Here's how the part is built. I have some questions about the finished solid (model axes, mm). Face numbers are marked on the shaded views. A direction names the side the tool comes from. Give positions to 0.01 mm unless a question says otherwise; leave off trailing zeros. Write each loop counter-clockwise with the first axis right and the second up, starting at its lowest first coordinate (ties: lowest second). Pieces come first, ordered by that corner, then holes. Notation, with made-up numbers: (76.5, 50) -> (127.5, 50) arc R25 ccw to (127.5, 84) -> close; hole circle Ø5 at (16.25, 58). An arc over 180 degrees is marked (long way). Use one line per item in the form item = value.
```python
from build123d import *

# Parameters (mm, degrees)
BOSS_EXTRUDE1_DEPTH = 3
SKETCH2_R           = 1.7
CUT_EXTRUDE1_DEPTH  = 3


with BuildPart() as part:
    # Sketch1 → Boss-Extrude1 (new body)
    with BuildSketch(Plane.XY):
        Polygon((10.5, 20.853495779), (-10.5, 20.853495779), (-10.5, 16.353495779), (-5.75, 16.353495779), (-5.75, -11.146504221), (5.75, -11.146504221), (5.75, 16.353495779), (10.5, 16.353495779), align=None)
    extrude(amount=BOSS_EXTRUDE1_DEPTH)

    # Sketch2 → Cut-Extrude1 (cut)
    with BuildSketch(Plane.XY.offset(3)):
        with Locations((0, -6.446504221)):
            Circle(SKETCH2_R)
        with BuildLine():
            Line((1.725328859, 12.62816692), (1.725328859, 9.078824638))
            ThreePointArc((1.725328859, 9.078824638), (0, 7.353495779), (-1.725328859, 9.078824638))
            Line((-1.725328859, 9.078824638), (-1.725328859, 12.62816692))
            ThreePointArc((-1.725328859, 12.62816692), (0, 14.353495779), (1.725328859, 12.62816692))
        make_face()
    extrude(amount=-CUT_EXTRUDE1_DEPTH, mode=Mode.SUBTRACT)


solid = part.part
```
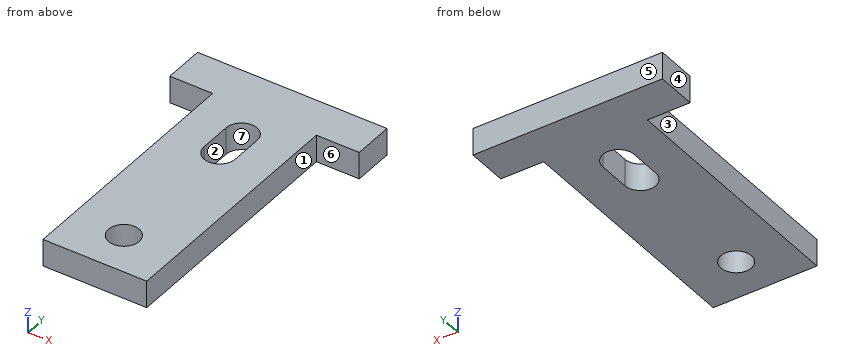
Q1. If I drill on line 1 along Y through (x, z) = (0, 1.15); line 2 along X through (y, z) = (9.5, 0.8); line 3 along X through (y, z) = (7, 1.15), over which ranges is the centre line in solid material (lowest first)? Write a range as from..to.
Result set:
line_1 = -11.15..-8.15, -4.75..7.35, 14.35..20.85
line_2 = -5.75..-1.73, 1.73..5.75
line_3 = -5.75..5.75
Q2. I want a section at C-C, the plane z = 2.15. Write out the boundary of the cut face in (x, y), and give its area (3 significant figures).
Result set:
outline = (-10.5, 16.35) -> (-5.75, 16.35) -> (-5.75, -11.15) -> (5.75, -11.15) -> (5.75, 16.35) -> (10.5, 16.35) -> (10.5, 20.85) -> (-10.5, 20.85) -> close; hole (-1.73, 9.08) arc R1.73 ccw to (1.73, 9.08) -> (1.73, 12.63) arc R1.73 ccw to (-1.73, 12.63) -> close; hole circle Ø3.4 at (0, -6.45)
area = 380 mm2
Q3. I want a section at A-A, the plane y = 10. Write out the boundary of the cut face in (x, z), and give its area (3 significant figures).
Result set:
outline = (-5.75, 0) -> (-1.73, 0) -> (-1.73, 3) -> (-5.75, 3) -> close; (1.73, 0) -> (5.75, 0) -> (5.75, 3) -> (1.73, 3) -> close
area = 24.1 mm2
Q4. I want a section at B-B, the plane x = 0. Write out the boundary of the cut face in (y, z), and give its area (3 significant figures).
Result set:
outline = (-11.15, 0) -> (-8.15, 0) -> (-8.15, 3) -> (-11.15, 3) -> close; (-4.75, 0) -> (7.35, 0) -> (7.35, 3) -> (-4.75, 3) -> close; (14.35, 0) -> (20.85, 0) -> (20.85, 3) -> (14.35, 3) -> close
area = 64.8 mm2
Q5. I want a section at D-D, the plane y = -5.5. Write out the boundary of the cut face in (x, z), and give its area (3 significant figures).
Result set:
outline = (-5.75, 0) -> (-1.41, 0) -> (-1.41, 3) -> (-5.75, 3) -> close; (1.41, 0) -> (5.75, 0) -> (5.75, 3) -> (1.41, 3) -> close
area = 26.0 mm2
Q6. Will these pins go through, and if not, where does the flat tip stop? pin 1 Ø1.5 at (y, z) = (7, 2) entering from +X; pin 2 Ø2 at (x, y) = (0, -6.45) entering from -Z.
Result set:
pin_1 = 5.75
pin_2 = through
Q7. If we mould it in two halves opening along Y, with no side actions, what happens to the marked faces 5, 6 and 7? For each: +Y half, -Y half, draft (parallel to the pull), parting line (faces both ways), or undercut.
Result set:
face_5 = +Y half
face_6 = -Y half
face_7 = undercut
Q8. Which directions (+Z, -Z, +X, -X, +Y, -Y) give clear straight access to the entire face, cutting with the end or side of a thin tool? Please do the marked faces 1, 2, 3 and 4.
Result set:
face_1 = +Z, -Z, +X, -Y
face_2 = +Z, -Z
face_3 = +Z, -Z, -X, -Y
face_4 = +Z, -Z, -X, +Y, -Y
